Autodesk Inventor part; units mm, degrees
ref_plane "YZ Plane" through (0, 0, 0) normal (1, 0, 0) x (0, 1, 0)
ref_plane "XZ Plane" through (0, 0, 0) normal (0, 1, 0) x (-1, 0, 0)
ref_plane "XY Plane" through (0, 0, 0) normal (0, 0, 1) x (1, 0, 0)
sketch "Esboço1" plane through (0, 0, 0) normal (0, 0, 1) x (1, 0, 0)
  line L0 (-20, -15) -> (20, -15)
  line L1 (25, -10) -> (25, 10)
  line L2 (20, 15) -> (-20, 15)
  line L3 (-25, 10) -> (-25, -10)
  line L4 (-25, -15) -> (25, 15) construction
  line L5 (10.842, 0) -> (-10.842, 0) construction
  line L6 (0, 2.6199) -> (0, -2.6199) construction
  line L7 (1.3987, 0) -> (-1.3987, 0) construction
  arc A0 (20, 15) -> (25, 10) centre (25, 15) ccw
  arc A1 (25, -10) -> (20, -15) centre (25, -15) ccw
  arc A2 (-25, 10) -> (-20, 15) centre (-25, 15) ccw
  arc A3 (-20, -15) -> (-25, -10) centre (-25, -15) ccw
  point P0 (0, 0)
  dimension "d0" = 30
  dimension "d1" = 50
  dimension "d22" = 10
  dimension "d23" = 5
  dimension "d24" = 5
extrude "Extrusão1" add sketch "Esboço1" along normal blind 20
sketch "Esboço2" plane through (-25, -10, 0) normal (-1, 0, 0) x (0, 0, 1)
  circle A0 centre (10, 8) radius 2.5
  line L0 (20, 20) -> (20, 0)
  line L1 (0, 0) -> (20, 0)
  circle A1 centre (10, 8) radius 3.5
  line L2 (10, 0) -> (10, 11.9886) construction
  line L3 (0, -5) -> (20, -5)
  point P0 (0, 10)
  dimension "d10" = 1
  dimension "d25" = 5
  dimension "d27" = 8
extrude "Extrusão2" add sketch "Esboço2" along normal blind 2
extrude "Extrusão3" add sketch "Esboço2" along normal blind 5 contours A0
fillet "Arredondamento1" radius 1 1 edges at (-27, -2, 6.5)
thread "Rosca1"
sketch "Esboço5" plane through (25, -10, 0) normal (1, 0, 0) x (0, 0, -1)
  line L0 (-20, 20) -> (0, 20)
  line L1 (0, 20) -> (0, 0)
  line L2 (0, 0) -> (-20, 0)
  line L3 (-20, 0) -> (-20, 20)
  line L4 (-15, 15) -> (-5, 15)
  line L5 (-5, 15) -> (-5, 5)
  line L6 (-5, 5) -> (-15, 5)
  line L7 (-15, 5) -> (-15, 15)
  point P0 (0, 10)
  dimension "d28" = 5
extrude "Extrusão4" add sketch "Esboço5" along normal blind 3 contours L4 L5 L6 L7
properties part number "receptor ftth fibra"
Here's how the part is built. I have some questions about the finished solid (model axes, mm). A direction names the side the tool comes from. Coordinates: 2 decimals unless noted, no trailing zeros. Loops run counter-clockwise (first coordinate to the right, second up) from the corner with the lowest first, then second, coordinate; pieces in that order, holes last. Notation, with made-up numbers: (16.5, 14) -> (56.5, 14) arc R24 cw to (56.5, 24) -> close; hole circle Ø11 at (43, 40.5). An arc over 180 degrees is marked (long way). Use one line per item in the form item = value. Start each with the question number.
(1) On a 3-axis mill with a long thin cutter (end or side, diameter ignored), from which of +Z, -Z, +X, -X, +Y, -Y can I reach the whole of each face in a straight line? I mean faces 1 (the face through (26, 0, 15)), 2 (the face through (-28.48, 0.44, 9.46)), 3 (the face through (26, 5, 10)), 4 (the face through (26, -5, 10)). Say none if no direction works.
(2) If we section it at C-C (z = 17): Please give me the cut outline in (x, y).
(3) Will these pins go through, and if not, where does the flat tip stop? pin 1 (5 mm diameter, centred on y = -11.5, z = 11.5, fed in from +X); pin 2 (3.5 mm diameter, centred on x = 26.5, z = 10, fed in from -Y); pin 3 (3.5 mm diameter, centred on x = 26.5, z = 8, fed in from +Y).
(4) Please list where these lines run through material, in increasing order: line 1 along X through (y, z) = (-6.5, 7.5); line 2 along X through (y, z) = (0, 5.5); line 3 along Y through (x, z) = (-22, 10.75).
(5) If we section it at D-D (x = 22.5): Please give me the cut outline in (y, z).
Verdict:
q1.face_1 = +Z, +X, +Y, -Y
q1.face_2 = -X
q1.face_3 = +Z, -Z, +X, +Y
q1.face_4 = +Z, -Z, +X, -Y
q2.outline = (-25, -10) arc R5 cw to (-20, -15) -> (20, -15) arc R5 cw to (25, -10) -> (25, 10) arc R5 cw to (20, 15) -> (-20, 15) arc R5 cw to (-25, 10) -> close
q3.pin_1 = 25
q3.pin_2 = -10.01
q3.pin_3 = 10.01
q4.line_1 = -25 to 25
q4.line_2 = -25 to 28
q4.line_3 = -11 to 11
q5.outline = (-10.67, 0) -> (10.67, 0) -> (10.67, 20) -> (-10.67, 20) -> close
